Work out the finished part from the listing and answer in its coordinate system (mm). A direction names the side the tool comes from. Round coordinates to 2 decimals unless told otherwise and drop trailing zeros. Order: outer loops, then holes, each group sorted by start corner. A loop starts at its lowest first (then second) coordinate and runs counter-clockwise, first axis right, second up.
from build123d import *

# Parameters (mm, degrees)
SKETCH1_W             = 80
SKETCH1_H             = 225
BOSS_EXTRUDE1_DEPTH   = 29
CUT_EXTRUDE1_REACH    = 124.871
SKETCH3_R             = 8
CUT_EXTRUDE2_DEPTH    = 20
M8_TAPPED_HOLE1_D     = 6.8
M8_TAPPED_HOLE1_DEPTH = 19.75
M8_TAPPED_HOLE1_TIP   = 2.042926105
CUT_EXTRUDE3_REACH    = 124.871
SKETCH15_W            = 12
SKETCH15_H            = 11.5
SKETCH16_R            = 8.5
CUT_EXTRUDE4_DEPTH    = 5
CUT_EXTRUDE5_REACH    = 124.871
SKETCH17_R            = 4


with BuildPart() as part:
    # Sketch1 → Boss-Extrude1 (new body)
    with BuildSketch(Plane(origin=(0, 0, 0), x_dir=(1, 0, 0), z_dir=(0, 1, 0))):
        Rectangle(SKETCH1_W, SKETCH1_H)
    extrude(amount=-BOSS_EXTRUDE1_DEPTH)

    # Sketch2 → Cut-Extrude1 (cut, up to next)
    with BuildSketch(Plane(origin=(0, 0, 0), x_dir=(1, 0, 0), z_dir=(0, 1, 0)), mode=Mode.PRIVATE) as cut_extrude1_sk1:
        with BuildLine():
            Line((30.5, 72.87), (30.5, 95.77))
            ThreePointArc((30.5, 95.77), (33, 98.27), (35.5, 95.77))
            Line((35.5, 95.77), (35.5, 72.87))
            ThreePointArc((35.5, 72.87), (33, 70.37), (30.5, 72.87))
        make_face()
    cut_extrude1_tool1 = extrude(cut_extrude1_sk1.sketch, amount=-CUT_EXTRUDE1_REACH, mode=Mode.PRIVATE) & part.part
    # Sketch2 → Cut-Extrude1 (cut, up to next)
    with BuildSketch(Plane(origin=(0, 0, 0), x_dir=(1, 0, 0), z_dir=(0, 1, 0)), mode=Mode.PRIVATE) as cut_extrude1_sk2:
        with BuildLine():
            Line((30.5, 33.86), (30.5, 48.36))
            ThreePointArc((30.5, 48.36), (33, 50.86), (35.5, 48.36))
            Line((35.5, 48.36), (35.5, 33.86))
            ThreePointArc((35.5, 33.86), (33, 31.36), (30.5, 33.86))
        make_face()
    cut_extrude1_tool2 = extrude(cut_extrude1_sk2.sketch, amount=-CUT_EXTRUDE1_REACH, mode=Mode.PRIVATE) & part.part
    # Sketch2 → Cut-Extrude1 (cut, up to next)
    with BuildSketch(Plane(origin=(0, 0, 0), x_dir=(1, 0, 0), z_dir=(0, 1, 0)), mode=Mode.PRIVATE) as cut_extrude1_sk3:
        with BuildLine():
            Line((31.5, -47.14), (31.5, -18.14))
            ThreePointArc((31.5, -18.14), (31.207106781, -17.432893219), (30.5, -17.14))
            Line((30.5, -17.14), (-7.5, -17.14))
            ThreePointArc((-7.5, -17.14), (-8.207106781, -17.432893219), (-8.5, -18.14))
            Line((-8.5, -18.14), (-8.5, -47.14))
            ThreePointArc((-8.5, -47.14), (-7.035533906, -50.675533906), (-3.5, -52.14))
            Line((-3.5, -52.14), (26.5, -52.14))
            ThreePointArc((26.5, -52.14), (30.035533906, -50.675533906), (31.5, -47.14))
        make_face()
    cut_extrude1_tool3 = extrude(cut_extrude1_sk3.sketch, amount=-CUT_EXTRUDE1_REACH, mode=Mode.PRIVATE) & part.part
    # Sketch2 → Cut-Extrude1 (cut, up to next)
    with BuildSketch(Plane(origin=(0, 0, 0), x_dir=(1, 0, 0), z_dir=(0, 1, 0)), mode=Mode.PRIVATE) as cut_extrude1_sk4:
        with BuildLine():
            Line((30.5, -95.77), (30.5, -72.87))
            ThreePointArc((30.5, -72.87), (33, -70.37), (35.5, -72.87))
            Line((35.5, -72.87), (35.5, -95.77))
            ThreePointArc((35.5, -95.77), (33, -98.27), (30.5, -95.77))
        make_face()
    cut_extrude1_tool4 = extrude(cut_extrude1_sk4.sketch, amount=-CUT_EXTRUDE1_REACH, mode=Mode.PRIVATE) & part.part
    add(cut_extrude1_tool1.solids().sort_by_distance((33, 0, -84.32))[0], mode=Mode.SUBTRACT)
    add(cut_extrude1_tool2.solids().sort_by_distance((33, 0, -41.11))[0], mode=Mode.SUBTRACT)
    add(cut_extrude1_tool3.solids().sort_by_distance((11.5, 0, 34.518764))[0], mode=Mode.SUBTRACT)
    add(cut_extrude1_tool4.solids().sort_by_distance((33, 0, 84.32))[0], mode=Mode.SUBTRACT)

    # Sketch3 → Cut-Extrude2 (cut)
    with BuildSketch(Plane(origin=(0, 0, 0), x_dir=(1, 0, 0), z_dir=(0, 1, 0))):
        with Locations(Location((15, 72.5, 0), (0, 0, 270))):
            Circle(SKETCH3_R)
        with Locations(Location((15, 41.11, 0), (0, 0, 270))):
            Circle(SKETCH3_R)
        with Locations(Location((15, -7, 0), (0, 0, 270))):
            Circle(SKETCH3_R)
        with Locations(Location((15, -72.5, 0), (0, 0, 270))):
            Circle(SKETCH3_R)
        with Locations(Location((-20, -72.5, 0), (0, 0, 270))):
            Circle(SKETCH3_R)
        with Locations(Location((-20, -7, 0), (0, 0, 270))):
            Circle(SKETCH3_R)
        with Locations(Location((-20, 41.11, 0), (0, 0, 270))):
            Circle(SKETCH3_R)
        with Locations(Location((-20, 72.5, 0), (0, 0, 270))):
            Circle(SKETCH3_R)
    extrude(amount=-CUT_EXTRUDE2_DEPTH, mode=Mode.SUBTRACT)

    # M8 Tapped Hole1
    with Locations(Plane(origin=(0, 0, 0), x_dir=(1, 0, 0), z_dir=(0, 1, 0))):
        with Locations((-25, -36), (20, 22), (-2.5, 72.5), (-2.5, -72.5)):
            Hole(M8_TAPPED_HOLE1_D / 2, depth=M8_TAPPED_HOLE1_DEPTH)
            with Locations((0, 0, -(M8_TAPPED_HOLE1_DEPTH + M8_TAPPED_HOLE1_TIP / 2))):  # 118° drill point
                Cone(0, M8_TAPPED_HOLE1_D / 2, M8_TAPPED_HOLE1_TIP, mode=Mode.SUBTRACT)

    # Sketch15 → Cut-Extrude3 (cut, up to next)
    with BuildSketch(Plane(origin=(0, 0, 0), x_dir=(1, 0, 0), z_dir=(0, 1, 0)), mode=Mode.PRIVATE) as cut_extrude3_sk1:
        with Locations((34.75, -106.75)):
            Rectangle(SKETCH15_W, SKETCH15_H)
    cut_extrude3_tool1 = extrude(cut_extrude3_sk1.sketch, amount=-CUT_EXTRUDE3_REACH, mode=Mode.PRIVATE) & part.part
    add(cut_extrude3_tool1.solids().sort_by_distance((34.75, 0, 106.75))[0], mode=Mode.SUBTRACT)

    # Sketch16 → Cut-Extrude4 (cut)
    with BuildSketch(Plane.XZ.offset(29)):
        with Locations(Location((11.5, 100, 0), (0, 0, 270))):
            Circle(SKETCH16_R)
        with Locations(Location((11.5, -100, 0), (0, 0, 270))):
            Circle(SKETCH16_R)
    extrude(amount=-CUT_EXTRUDE4_DEPTH, mode=Mode.SUBTRACT)

    # Sketch17 → Cut-Extrude5 (cut, up to next)
    with BuildSketch(Plane(origin=(0, 0, 0), x_dir=(1, 0, 0), z_dir=(0, 1, 0)), mode=Mode.PRIVATE) as cut_extrude5_sk1:
        with Locations(Location((11.5, 9.86, 0), (0, 0, 270))):
            Circle(SKETCH17_R)
    cut_extrude5_tool1 = extrude(cut_extrude5_sk1.sketch, amount=-CUT_EXTRUDE5_REACH, mode=Mode.PRIVATE) & part.part
    add(cut_extrude5_tool1.solids().sort_by_distance((11.5, 0, -9.86))[0], mode=Mode.SUBTRACT)


solid = part.part
Item 1: Find section B-B (y = -26). State how many separate pieces and enclosed holes the cut face has, plus the area to 3 significant figures.
Item 2: Find section A-A (z = -9.86). Write down the section's boundary in (x, y).
Item 3: Find the intervals of material crossed by line 1 along X through (y, z) = (-5.5, 72.5); line 2 along X through (y, z) = (-5, 7); line 3 along X through (y, z) = (-26.5, 73), in increasing order.
Item 4: Find section C-C (z = -41.11). Write down the section's boundary in (x, y), plus the area to 4 significant figures.
Item 5: Given pin 1 (5 mm diameter, centred on x = -20.5, z = 73, fed in from +Y); pin 2 (9 mm diameter, centred on x = 33.5, y = -17.5, fed in from +Z); pin 3 (5 mm diameter, centred on x = 8, z = 102.5, fed in from -Y), each flat-ended and moving along its own axis, determine where each tip first touches the part or whether it passes through.
Item 6: For a pull along X with two mould halves and no side action, classify faces 1 (the face through (28.75, -14, 107)), 2 (the face through (-20, -20, -41)), 3 (the face through (-1, -29, -2)) as released by +X, released by -X, zero draft, split by the parting line, or undercut.
Item 7: A tool of negligible diameter and unlimited length cuts with its end or side. For faces 4 (the face through (35.5, -14, 84)), 5 (the face through (15, -20, -41)), from which of +Z, -Z, +X, -X, +Y, -Y can it reach the whole face along a straight path? Write none if from no direction.
Model answer:
1. separate pieces: 1
1. enclosed holes: 7
1. area: 15,600 mm2
2. outline: (-40, -29) - (7.5, -29) - (7.5, 0) - (-40, 0) - close; (15.5, -29) - (40, -29) - (40, 0) - (15.5, 0) - close
3. line 1: x = -40 to -28, -12 to -5.9, 0.9 to 7, 23 to 30.53, 35.47 to 40
3. line 2: x = -40 to -28, -12 to 7, 23 to 40
3. line 3: x = -40 to 30.5, 35.5 to 40
4. outline: (-40, -29) - (30.5, -29) - (30.5, 0) - (23, 0) - (23, -20) - (7, -20) - (7, 0) - (-12, 0) - (-12, -20) - (-28, -20) - (-28, 0) - (-40, 0) - close; (35.5, -29) - (40, -29) - (40, 0) - (35.5, 0) - close
4. area: 1,535 mm2
5. pin 1: stops at y = -20
5. pin 2: stops at z = 101
5. pin 3: stops at y = -24
6. face 1: released by +X
6. face 2: undercut
6. face 3: zero draft
7. face 4: +Y, -Y
7. face 5: +Y
